Can you work these out from the model? Positions are in its coordinate system, mm. Round coordinates to 2 decimals unless told otherwise and drop trailing zeros. Loops run counter-clockwise (first coordinate to the right, second up) from the corner with the lowest first, then second, coordinate; pieces in that order, holes last. Notation, with made-up numbers: (-35.5, -29) -> (-8.5, -29) arc R27 cw to (-8.5, -5) -> close; hole circle Ø8 at (33, 34.5). An arc over 180 degrees is marked (long way). Answer as a JSON object with one key per item and string values.
```python
from build123d import *

# Parameters (mm, degrees)
SKETCH1_R           = 13.75
SKETCH1_R_2         = 7.62
BOSS_EXTRUDE1_DEPTH = 7
CUT_EXTRUDE1_REACH  = 9
SKETCH3_R           = 1.9499961


with BuildPart() as part:
    # Sketch1 → Boss-Extrude1 (new body)
    with BuildSketch(Plane.XY):
        Circle(SKETCH1_R)
        Circle(SKETCH1_R_2, mode=Mode.SUBTRACT)
    extrude(amount=-BOSS_EXTRUDE1_DEPTH)

    # Sketch3 → Cut-Extrude1 (cut, up to next)
    with BuildSketch(Plane.XY, mode=Mode.PRIVATE) as cut_extrude1_sk1:
        with Locations((-11.49999986, 0)):
            Circle(SKETCH3_R)
    cut_extrude1_tool1 = extrude(cut_extrude1_sk1.sketch, amount=-CUT_EXTRUDE1_REACH, mode=Mode.PRIVATE) & part.part
    add(cut_extrude1_tool1.solids().sort_by_distance((-11.5, 0, 0))[0], mode=Mode.SUBTRACT)
    # Sketch3 → Cut-Extrude1 (cut, up to next)
    with BuildSketch(Plane.XY, mode=Mode.PRIVATE) as cut_extrude1_sk2:
        with Locations((0, 11.49999986)):
            Circle(SKETCH3_R)
    cut_extrude1_tool2 = extrude(cut_extrude1_sk2.sketch, amount=-CUT_EXTRUDE1_REACH, mode=Mode.PRIVATE) & part.part
    add(cut_extrude1_tool2.solids().sort_by_distance((0, 11.5, 0))[0], mode=Mode.SUBTRACT)
    # Sketch3 → Cut-Extrude1 (cut, up to next)
    with BuildSketch(Plane.XY, mode=Mode.PRIVATE) as cut_extrude1_sk3:
        with Locations((11.49999986, 0)):
            Circle(SKETCH3_R)
    cut_extrude1_tool3 = extrude(cut_extrude1_sk3.sketch, amount=-CUT_EXTRUDE1_REACH, mode=Mode.PRIVATE) & part.part
    add(cut_extrude1_tool3.solids().sort_by_distance((11.5, 0, 0))[0], mode=Mode.SUBTRACT)
    # Sketch3 → Cut-Extrude1 (cut, up to next)
    with BuildSketch(Plane.XY, mode=Mode.PRIVATE) as cut_extrude1_sk4:
        with Locations((0, -11.49999986)):
            Circle(SKETCH3_R)
    cut_extrude1_tool4 = extrude(cut_extrude1_sk4.sketch, amount=-CUT_EXTRUDE1_REACH, mode=Mode.PRIVATE) & part.part
    add(cut_extrude1_tool4.solids().sort_by_distance((0, -11.5, 0))[0], mode=Mode.SUBTRACT)


solid = part.part
```
Q1. I want a section at D-D, the plane x = 11.5. Write out the boundary of the cut face in (y, z).
Determined:
{"outline": "(-7.54, -7) -> (-1.95, -7) -> (-1.95, 0) -> (-7.54, 0) -> close; (1.95, -7) -> (7.54, -7) -> (7.54, 0) -> (1.95, 0) -> close"}
Q2. I want a section at B-B, the plane z = -2.75. Write out the boundary of the cut face in (x, y), then the cut area to 3 significant figures.
Determined:
{"outline": "circle Ø27.5 at (0, 0); hole circle Ø3.9 at (-11.5, 0); hole circle Ø15.24 at (0, 0); hole circle Ø3.9 at (0, -11.5); hole circle Ø3.9 at (0, 11.5); hole circle Ø3.9 at (11.5, 0)", "area": "364 mm²"}
Q3. I'm going to push flat-ended pins straight in: pin 1 (1.5 mm diameter, centred on y = -7.5, z = -2, fed in from -X); pin 2 (4 mm diameter, centred on x = 1, y = 5, fed in from -Z); pin 3 (3 mm diameter, centred on x = 2, z = -3.5, fed in from -Y); pin 4 (1.5 mm diameter, centred on x = -7.5, z = -5, fed in from +Y). Where does each tip first touch, or does it pass through?
Determined:
{"pin 1": "x = -11.98", "pin 2": "through", "pin 3": "y = -13.74", "pin 4": "y = 11.98"}
Q4. I want a section at A-A, the plane x = 0. Write out the boundary of the cut face in (y, z), then the cut area to 3 significant figures.
Determined:
{"outline": "(-13.75, -7) -> (-13.45, -7) -> (-13.45, 0) -> (-13.75, 0) -> close; (-9.55, -7) -> (-7.62, -7) -> (-7.62, 0) -> (-9.55, 0) -> close; (7.62, -7) -> (9.55, -7) -> (9.55, 0) -> (7.62, 0) -> close; (13.45, -7) -> (13.75, -7) -> (13.75, 0) -> (13.45, 0) -> close", "area": "31.2 mm²"}
Q5. We'd pull the mould along X, two halves only. Please class faces 1 (the flat face through (6, -6, 0)), 2 (the cylindrical face through (-0.254, 13.433, -3.451)), 3 (the cylindrical face through (-2.981, -13.423, -3.451)): pulls with the +X half, pulls with the -X half, needs draft (parallel to the pull), parting line crosses it, or undercut.
Determined:
{"face 1": "needs draft", "face 2": "undercut", "face 3": "parting line crosses it"}
Q6. If I drill on L1, parallel to Y at x = 0, z = -3; L2, parallel to X at y = -1, z = -3.5; L3, parallel to Y at x = -5.5, z = -0.25, over which ranges is the centre line in solid material (lowest first)? Write a range as [from, to].
Determined:
{"L1": "[-13.75, -13.45], [-9.55, -7.62], [7.62, 9.55], [13.45, 13.75]", "L2": "[-13.71, -13.17], [-9.83, -7.55], [7.55, 9.83], [13.17, 13.71]", "L3": "[-12.6, -5.27], [5.27, 12.6]"}
